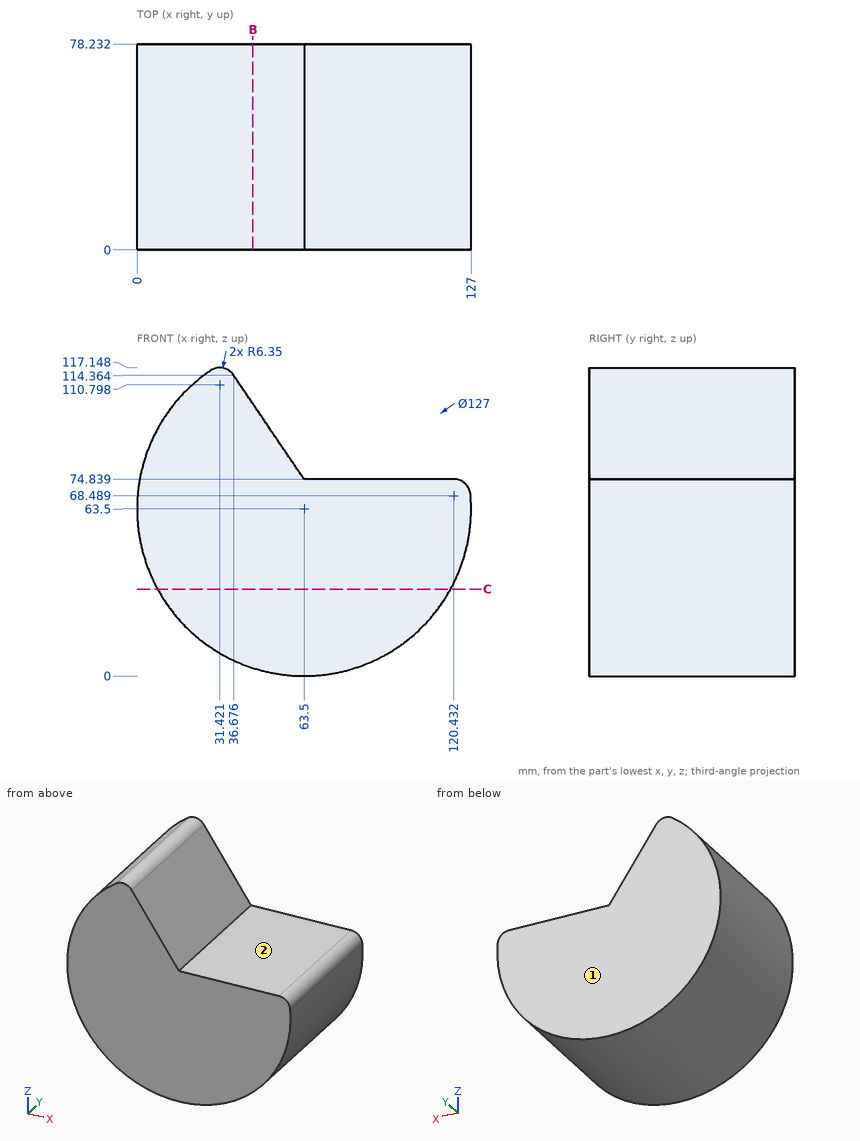
Study the drawing (mm; zero at the part's minimum x, y, z) and answer. A direction names the side the tool comes from. Coordinates: 2 decimals unless noted, no trailing zeros. Write each loop counter-clockwise with the first axis right and the second up, starting at its lowest first coordinate (ties: lowest second). Pieces come first, ordered by that corner, then holes. Notation, with made-up numbers: (-27, 27.5) - (22, 27.5) arc R20 ccw to (22, 61.5) - close; hole circle Ø6 at (-13, 37). An arc over 180 degrees is marked (long way). Put each result on its own line as item: value.
1. A tool of negligible diameter and unlimited length cuts with its end or side. For the marked faces 1 and 2, from which of +Z, -Z, +X, -X, +Y, -Y can it reach the whole face along a straight path? Write none if from no direction.
Answer sheet:
face 1: +Z, -Z, +X, -X, +Y
face 2: +Z, +X, +Y, -Y
2. The part is cut by section B-B on x = 44. Give the vertices of the cut face in (y, z), plus the area to 3 significant figures.
Answer sheet:
outline: (0, 3.07) - (78.23, 3.07) - (78.23, 103.57) - (0, 103.57) - close
area: 7,860 mm^2
3. Flat-ended cylindrical pins translate along their axes: pin 1 Ø2 at (x, y) = (63, 62.5) entering from -Z; pin 2 Ø1.5 at (x, y) = (103, 67.5) entering from -Z (1 decimal); pin 3 Ø1.5 at (y, z) = (11, 82) entering from +X. Find the tip coordinate at first contact, or state that the pin passes through.
Answer sheet:
pin 1: stops at z = 0
pin 2: stops at z = 13.2
pin 3: stops at x = 59.15
4. The part is cut by section C-C on z = 33. Give the vertices of the cut face in (x, y) (1 decimal), plus the area to 3 significant figures.
Answer sheet:
outline: (7.8, 0) - (119.2, 0) - (119.2, 78.2) - (7.8, 78.2) - close
area: 8,710 mm^2
5. Find the intervals of material crossed by line 1 along Z through (x, y) = (43, 70.5) (1 decimal); line 2 along Z through (x, y) = (81, 10.5); line 3 along X through (y, z) = (21, 78.5) (1 decimal), in increasing order. Write a range as from..to.
Answer sheet:
line 1: z = 3.4..105
line 2: z = 2.46..74.84
line 3: x = 1.8..61
